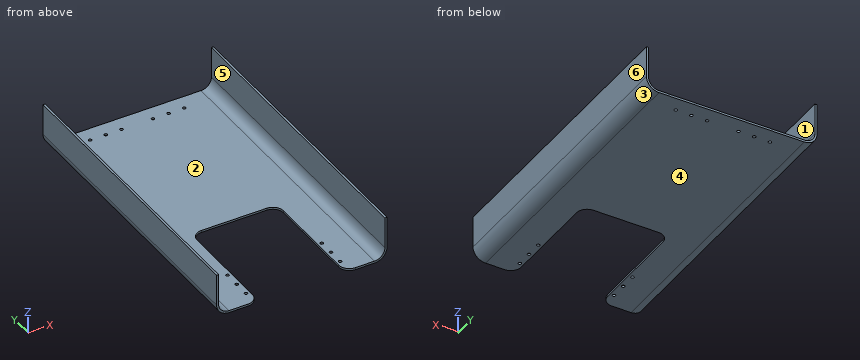
from build123d import *

# Parameters (mm, degrees)
EXTRUDE_THIN1_DEPTH     = 564
CUT_EXTRUDE2_DEPTH      = 594.060705156
CUT_EXTRUDE2_DEPTH_BACK = 594.060705156
SKETCH3_W               = 165
SKETCH3_H               = 220
FILLET1_R               = 20
SKETCH4_R               = 3
CUT_EXTRUDE3_DEPTH      = 594.060705156


with BuildPart() as part:
    # Sketch1 → Extrude-Thin1 (new body)
    with BuildSketch(Plane(origin=(0, 0, 0), x_dir=(1, 0, 0), z_dir=(0, 1, 0))):
        with BuildLine():
            Line((-159, -80), (-159, -20))
            ThreePointArc((-159, -20), (-153.142135624, -5.857864376), (-139, 0))
            Line((-139, 0), (139, 0))
            ThreePointArc((139, 0), (153.142135624, -5.857864376), (159, -20))
            Line((159, -20), (159, -80))
            Line((159, -80), (163, -80))
            Line((163, -80), (163, -20))
            ThreePointArc((163, -20), (155.970562748, -3.029437252), (139, 4))
            Line((139, 4), (-139, 4))
            ThreePointArc((-139, 4), (-155.970562748, -3.029437252), (-163, -20))
            Line((-163, -20), (-163, -80))
            Line((-163, -80), (-159, -80))
        make_face()
    extrude(amount=EXTRUDE_THIN1_DEPTH)

    # Sketch3 → Cut-Extrude2 (cut, two sides: drawn at the far end of the back side and taken through both)
    with BuildSketch(Plane(origin=(0, 0, -4), x_dir=(-1, 0, 0), z_dir=(0, 0, -1)).offset(-CUT_EXTRUDE2_DEPTH_BACK)):
        with Locations((0, 110)):
            Rectangle(SKETCH3_W, SKETCH3_H)
    extrude(amount=CUT_EXTRUDE2_DEPTH + CUT_EXTRUDE2_DEPTH_BACK, mode=Mode.SUBTRACT)

    # Fillet1
    fillet1_edges = [part.edges().sort_by_distance(p)[0] for p in [
        (-82.5, 0, -2),
        (82.5, 0, -2),
        (82.5, 220, -2),
        (-82.5, 220, -2),
    ]]
    fillet(fillet1_edges, radius=FILLET1_R)

    # Sketch4 → Cut-Extrude3 (cut, through all)
    with BuildSketch(Plane(origin=(0, 0, -4), x_dir=(-1, 0, 0), z_dir=(0, 0, -1))):
        with Locations((-90, 535)):
            Circle(SKETCH4_R)
        with Locations((-60, 535)):
            Circle(SKETCH4_R)
        with Locations((-30, 535)):
            Circle(SKETCH4_R)
        with Locations((-90, 88.126)):
            Circle(SKETCH4_R)
        with Locations((-90, 58.126)):
            Circle(SKETCH4_R)
        with Locations((-90, 28.126)):
            Circle(SKETCH4_R)
    cut_extrude3 = extrude(amount=-CUT_EXTRUDE3_DEPTH, mode=Mode.SUBTRACT)

    # Mirror1: Cut-Extrude3 across plane
    add(cut_extrude3.mirror(Plane(origin=(0, 0, 0), x_dir=(0, 0, 1), z_dir=(1, 0, 0))), mode=Mode.SUBTRACT)


solid = part.part
Work out the finished part from the listing and answer in its coordinate system (mm). Face numbers are marked on the shaded views. A direction names the side the tool comes from. Round coordinates to 2 decimals unless told otherwise and drop trailing zeros. Write each loop counter-clockwise with the first axis right and the second up, starting at its lowest first coordinate (ties: lowest second). Pieces come first, ordered by that corner, then holes.
1) A cutting plane is placed at D-D (x = -108.5). Give the vertices of the cut face in (y, z).
2) A cutting plane is placed at B-B (y = 317.5). Give the vertices of the cut face in (x, z), plus the area to 3 significant figures.
3) A cutting plane is placed at C-C (x = 2). Give the vertices of the cut face in (y, z).
4) Straight lines are drawn through the part: line 1 (X direction, y = 306.5, z = 47); line 2 (Y direction, x = -90, z = -3); line 3 (Y direction, x = 30, z = -1.6). For each, find the intervals that lie inside material, in ascending order.
5) A tool of negligible diameter and unlimited length cuts with its end or side. For the marked faces 5 and 6, from which of +Z, -Z, +X, -X, +Y, -Y can it reach the whole face along a straight path? Write none if from no direction.
6) Given pin 1 Ø3.5 at (x, y) = (-90, 28.126) entering from +Z; pin 2 Ø2 at (x, z) = (-12, -1.5) entering from -Y; pin 3 Ø1 at (x, y) = (49, 290.5) entering from +Z; pin 4 Ø4.5 at (y, z) = (124, -2) entering from +X, each flat-ended and moving along its own axis, determine where each tip first touches the part or whether it passes through.
7) The mould has two halves that part along X. Classify the marked faces 1, 2, 3 and 4: pulls with the +X half, pulls with the -X half, needs draft (parallel to the pull), parting line crosses it, or undercut.
8) A cutting plane is placed at A-A (z = 60.5). Give the vertices of the cut face in (x, y), plus the area to 3 significant figures.
Completed:
1. outline: (0, -4) - (564, -4) - (564, 0) - (0, 0) - close
2. outline: (-163, 20) arc R24 ccw to (-139, -4) - (139, -4) arc R24 ccw to (163, 20) - (163, 80) - (159, 80) - (159, 20) arc R20 cw to (139, 0) - (-139, 0) arc R20 cw to (-159, 20) - (-159, 80) - (-163, 80) - close
2. area: 1,870 mm2
3. outline: (220, -4) - (564, -4) - (564, 0) - (220, 0) - close
4. line 1: x = -163 to -159, 159 to 163
4. line 2: y = 4.39 to 25.13, 31.13 to 55.13, 61.13 to 85.13, 91.13 to 532, 538 to 564
4. line 3: y = 220 to 532, 538 to 564
5. face 5: +Z, +Y, -Y
5. face 6: +Z, -Z, +X, +Y, -Y
6. pin 1: passes through
6. pin 2: stops at y = 220
6. pin 3: stops at z = 0
6. pin 4: stops at x = 152.64
7. face 1: undercut
7. face 2: undercut
7. face 3: pulls with the +X half
7. face 4: needs draft
8. outline: (-163, 0) - (-159, 0) - (-159, 564) - (-163, 564) - close; (159, 0) - (163, 0) - (163, 564) - (159, 564) - close
8. area: 4,510 mm2
